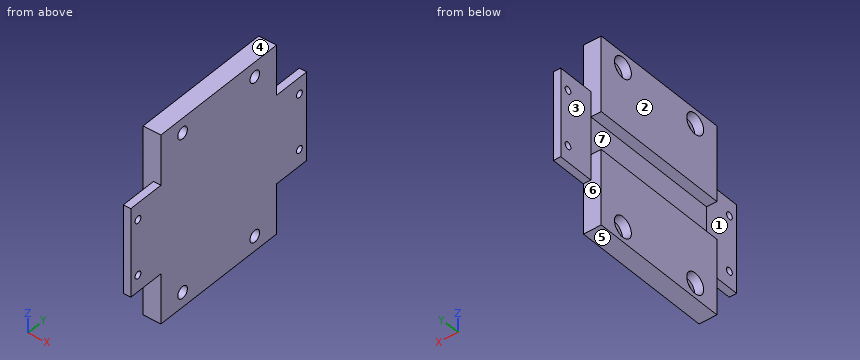
from build123d import *

# Parameters (mm, degrees)
SKETCH_1_W          = 32
SKETCH_1_H          = 24
EXTRUDE_1_DEPTH     = 3
SKETCH_4_W          = 6.4
SKETCH_4_H          = 24
CUT_EXTRUDE_1_DEPTH = 1.75
SKETCH_5_W          = 1.250005523
SKETCH_5_H          = 15
EXTRUDE_2_DEPTH     = 6.25
EXTRUDE_START       = -24
SKETCH_5_2_W        = 1.250005523
SKETCH_5_2_H        = 15
EXTRUDE_3_DEPTH     = 6.25
SKETCH_6_R          = 0.6
CUT_EXTRUDE_2_DEPTH = 25.455316395
SKETCH_7_R          = 1.75
SKETCH_7_R_2        = 1
CUT_EXTRUDE_4_DEPTH = 1.5
SKETCH_7_2_R        = 1
CUT_EXTRUDE_5_DEPTH = 25.455316395


with BuildPart() as part:
    # 草图1 → 凸台-拉伸1 (new body)
    with BuildSketch(Plane(origin=(0, 0, 0), x_dir=(0, 0, -1), z_dir=(1, 0, 0))):
        Rectangle(SKETCH_1_W, SKETCH_1_H)
    extrude(amount=EXTRUDE_1_DEPTH)

    # 草图4 → 切除-拉伸1 (cut)
    with BuildSketch(Plane.ZY):
        Rectangle(SKETCH_4_W, SKETCH_4_H)
    extrude(amount=-CUT_EXTRUDE_1_DEPTH, mode=Mode.SUBTRACT)

    # 草图5 → 凸台-拉伸2 (add)
    with BuildSketch(Plane.XZ.offset(12)):
        with Locations((2.374997239, 0)):
            Rectangle(SKETCH_5_W, SKETCH_5_H)
    extrude(amount=EXTRUDE_2_DEPTH)

    # 草图5<2> → 凸台-拉伸3 (add)
    with BuildSketch(Plane.XZ.offset(12).offset(EXTRUDE_START)):
        with Locations((2.374997239, 0)):
            Rectangle(SKETCH_5_2_W, SKETCH_5_2_H)
    extrude(amount=-EXTRUDE_3_DEPTH)

    # 草图6 → 切除-拉伸2 (cut, through all)
    with BuildSketch(Plane(origin=(3, 0, 0), x_dir=(0, 0, -1), z_dir=(1, 0, 0))):
        with Locations((4.695742753, -16.75)):
            Circle(SKETCH_6_R)
        with Locations((-4.695742753, -16.75)):
            Circle(SKETCH_6_R)
        with Locations((4.695742753, 16.75)):
            Circle(SKETCH_6_R)
        with Locations((-4.695742753, 16.75)):
            Circle(SKETCH_6_R)
    extrude(amount=-CUT_EXTRUDE_2_DEPTH, mode=Mode.SUBTRACT)

    # 草图7 → 切除-拉伸4 (cut)
    # profile 1 of 4: a face of its own
    with BuildSketch(Plane.ZY):
        with Locations((13.5, 7.5)):
            Circle(SKETCH_7_R)
        with Locations((13.5, 7.5)):
            Circle(SKETCH_7_R_2, mode=Mode.SUBTRACT)
    # profile 2 of 4: a face of its own
    with BuildSketch(Plane.ZY):
        with Locations((13.5, -7.5)):
            Circle(SKETCH_7_R)
        with Locations((13.5, -7.5)):
            Circle(SKETCH_7_R_2, mode=Mode.SUBTRACT)
    # profile 3 of 4: a face of its own
    with BuildSketch(Plane.ZY):
        with Locations((-13.5, 7.5)):
            Circle(SKETCH_7_R)
        with Locations((-13.5, 7.5)):
            Circle(SKETCH_7_R_2, mode=Mode.SUBTRACT)
    # profile 4 of 4: a face of its own
    with BuildSketch(Plane.ZY):
        with Locations((-13.5, -7.5)):
            Circle(SKETCH_7_R)
        with Locations((-13.5, -7.5)):
            Circle(SKETCH_7_R_2, mode=Mode.SUBTRACT)
    extrude(amount=-CUT_EXTRUDE_4_DEPTH, mode=Mode.SUBTRACT)

    # 草图7<2> → 切除-拉伸5 (cut, through all)
    with BuildSketch(Plane.ZY):
        with Locations((13.5, 7.5)):
            Circle(SKETCH_7_2_R)
        with Locations((13.5, -7.5)):
            Circle(SKETCH_7_2_R)
        with Locations((-13.5, -7.5)):
            Circle(SKETCH_7_2_R)
        with Locations((-13.5, 7.5)):
            Circle(SKETCH_7_2_R)
    extrude(amount=-CUT_EXTRUDE_5_DEPTH, mode=Mode.SUBTRACT)


solid = part.part
Could you check a few things on this model? Use its own coordinates, in mm. Face numbers are marked on the shaded views. A direction names the side the tool comes from. Give positions to 0.01 mm unless a question says otherwise; leave off trailing zeros. Write each loop counter-clockwise with the first axis right and the second up, starting at its lowest first coordinate (ties: lowest second). Pieces come first, ordered by that corner, then holes. Notation, with made-up numbers: (-13, 56) -> (3, 56) arc R24 cw to (3, 68) -> close; hole circle Ø1 at (-34, 83). An arc over 180 degrees is marked (long way). Write each question's results on one line, items separated by ' | '. Start each with the question number.
Q1. I'm going to push flat-ended pins straight in: pin 1 Ø1 at (y, z) = (-8, 12.5) entering from -X; pin 2 Ø3 at (y, z) = (-7.5, -14) entering from -X; pin 3 Ø2 at (y, z) = (14, -1) entering from -X. Where does each tip first touch, or does it pass through?
Q2. We'd pull the mould along Z, two halves only. Please class the marked faces 4, 5, 6 and 7: +Z half, -Z half, draft (parallel to the pull), parting line (faces both ways), or undercut.
Q3. I need wall thicknesses on probe 1 along Y at (x, z) = (0.5, 13.5); probe 2 along Y at (x, z) = (2.2, 13.5); probe 3 along Z at (x, y) = (1.55, -1). Which ranges of each line are inside material? Lowest first, please.
Q4. Suppose I cut it at B-B, the plane y = -7.5. List the corners of the cut face in (x, z) for me, and give its area (3 significant figures).
Q5. Suppose I cut it at C-C, the plane z = -13.5. List the corners of the cut face in (x, y) for me.
Q6. Suppose I cut it at A-A, the plane x = 1. List the corners of the cut face in (y, z) for me.
Q7. Which directions (+Z, -Z, +X, -X, +Y, -Y) give clear straight access to the entire face, cutting with the end or side of a thin tool? Please do the marked faces 1, 2 and 3.
Outcome:
1) pin 1: x = 1.5 | pin 2: x = 0 | pin 3: x = 1.75
2) face 4: +Z half | face 5: -Z half | face 6: draft | face 7: undercut
3) probe 1: -12 to -9.25, -5.75 to 5.75, 9.25 to 12 | probe 2: -12 to -8.5, -6.5 to 6.5, 8.5 to 12 | probe 3: -16 to -3.2, 3.2 to 16
4) outline: (0, -16) -> (3, -16) -> (3, -14.5) -> (1.5, -14.5) -> (1.5, -15.25) -> (0, -15.25) -> close; (0, -11.75) -> (1.5, -11.75) -> (1.5, -12.5) -> (3, -12.5) -> (3, 12.5) -> (1.5, 12.5) -> (1.5, 11.75) -> (0, 11.75) -> (0, 3.2) -> (1.75, 3.2) -> (1.75, -3.2) -> (0, -3.2) -> close; (0, 15.25) -> (1.5, 15.25) -> (1.5, 14.5) -> (3, 14.5) -> (3, 16) -> (0, 16) -> close | area: 68.3 mm2
5) outline: (0, -12) -> (3, -12) -> (3, -8.5) -> (1.5, -8.5) -> (1.5, -9.25) -> (0, -9.25) -> close; (0, -5.75) -> (1.5, -5.75) -> (1.5, -6.5) -> (3, -6.5) -> (3, 6.5) -> (1.5, 6.5) -> (1.5, 5.75) -> (0, 5.75) -> close; (0, 9.25) -> (1.5, 9.25) -> (1.5, 8.5) -> (3, 8.5) -> (3, 12) -> (0, 12) -> close
6) outline: (-12, -16) -> (12, -16) -> (12, -3.2) -> (-12, -3.2) -> close; (-12, 3.2) -> (12, 3.2) -> (12, 16) -> (-12, 16) -> close; hole circle Ø3.5 at (-7.5, -13.5); hole circle Ø3.5 at (-7.5, 13.5); hole circle Ø3.5 at (7.5, -13.5); hole circle Ø3.5 at (7.5, 13.5)
7) face 1: +Z, -Z, -X, -Y | face 2: +Z, -Z, -X, +Y, -Y | face 3: +Z, -Z, -X, +Y
